from build123d import *

# Parameters (mm, degrees)
SKETCH1_W           = 38.1
SKETCH1_H           = 63.5
BOSS_EXTRUDE1_DEPTH = 36.5125
SKETCH2_W           = 34.925
SKETCH2_H           = 39.6875
CUT_EXTRUDE1_DEPTH  = 62.585998054
SKETCH3_R           = 4.445
CUT_EXTRUDE2_DEPTH  = 76.685633751
SKETCH4_R           = 11.684
CUT_EXTRUDE3_DEPTH  = 6.35
SKETCH6_R           = 14.2621
CUT_EXTRUDE5_DEPTH  = 6.35
SKETCH7_R           = 7.62
CUT_EXTRUDE6_DEPTH  = 71.44279705


with BuildPart() as part:
    # Sketch1 → Boss-Extrude1 (new, symmetric)
    with BuildSketch(Plane.XY):
        Rectangle(SKETCH1_W, SKETCH1_H)
    extrude(amount=BOSS_EXTRUDE1_DEPTH, both=True)

    # Sketch2 → Cut-Extrude1 (cut, through all)
    with BuildSketch(Plane(origin=(19.05, 0, 0), x_dir=(0, 0, -1), z_dir=(1, 0, 0))):
        with Locations((-19.05, 0)):
            Rectangle(SKETCH2_W, SKETCH2_H)
    extrude(amount=-CUT_EXTRUDE1_DEPTH, mode=Mode.SUBTRACT)

    # Sketch3 → Cut-Extrude2 (cut, through all)
    with BuildSketch(Plane(origin=(0, 31.75, 0), x_dir=(1, 0, 0), z_dir=(0, 1, 0))):
        with Locations(Location((0, -20.6375, 0), (0, 0, 270))):
            Circle(SKETCH3_R)
    extrude(amount=-CUT_EXTRUDE2_DEPTH, mode=Mode.SUBTRACT)

    # Sketch4 → Cut-Extrude3 (cut)
    with BuildSketch(Plane(origin=(0, 31.75, 0), x_dir=(1, 0, 0), z_dir=(0, 1, 0))):
        with Locations(Location((0, -20.6375, 0), (0, 0, 270))):
            Circle(SKETCH4_R)
    cut_extrude3 = extrude(amount=-CUT_EXTRUDE3_DEPTH, mode=Mode.SUBTRACT)

    # Sketch6 → Cut-Extrude5 (cut)
    with BuildSketch(Plane(origin=(0, 31.75, 0), x_dir=(1, 0, 0), z_dir=(0, 1, 0))):
        with Locations(Location((0, 20.9296, 0), (0, 0, 270))):
            Circle(SKETCH6_R)
    cut_extrude5 = extrude(amount=-CUT_EXTRUDE5_DEPTH, mode=Mode.SUBTRACT)

    # Mirror1: Cut-Extrude3, Cut-Extrude5 across plane
    add(cut_extrude3.mirror(Plane.ZX), mode=Mode.SUBTRACT)
    add(cut_extrude5.mirror(Plane.ZX), mode=Mode.SUBTRACT)

    # Sketch7 → Cut-Extrude6 (cut, through all)
    with BuildSketch(Plane(origin=(0, 25.4, 0), x_dir=(1, 0, 0), z_dir=(0, 1, 0))):
        with Locations(Location((0, 20.9296, 0), (0, 0, 270))):
            Circle(SKETCH7_R)
    extrude(amount=-CUT_EXTRUDE6_DEPTH, mode=Mode.SUBTRACT)


solid = part.part
CAD build for the part. Positions are in the model's coordinates, mm. A direction names the side the tool comes from. Give positions to 0.01 mm unless a question says otherwise; leave off trailing zeros. Order: outer loops, then holes, each group sorted by start corner. A loop starts at its lowest first (then second) coordinate and runs counter-clockwise, first axis right, second up. Notation, with made-up numbers: (64, 86) - (85, 86) arc R5 cw to (85, 95) - close; hole circle Ø10 at (-19, 65). An arc over 180 degrees is marked (long way). Write each question's results on one line, items separated by ' | '.
1. Saw through at C-C on x = 0. Count the separate pieces of the cut face and the enclosed holes in it, and give its area (3 significant figures).
Calculated:
separate pieces: 4 | enclosed holes: 0 | area: 1,720 mm2
2. Pull direction Y, two halves, no side cores. Call faces 1 (the face through (-0.3, 31.75, 8.6)), 2 (the face through (-8.678, -28.619, -32.248)), 3 (the face through (0, 19.844, 15)): released by +Y, released by -Y, zero draft, split by the parting line, or undercut.
Calculated:
face 1: released by +Y | face 2: zero draft | face 3: undercut
3. Pin check, flat tips, straight feed: pin 1 (14 mm diameter, centred on x = 0, z = 20.64, fed in from +Y); pin 2 (10.5 mm diameter, centred on x = 0.5, z = 18, fed in from -Y); pin 3 (3 mm diameter, centred on x = 9, z = 14, fed in from +Y); pin 4 (12 mm diameter, centred on x = 7, y = -12, fed in from +Z). Stop position of each tip, or through.
Calculated:
pin 1: stops at y = 25.4 | pin 2: stops at y = -25.4 | pin 3: stops at y = 31.75 | pin 4: stops at z = 1.59
4. Probe L1, parallel to Y at x = 2, z = 9; L2, parallel to Y at x = -2.5, z = 31; L3, parallel to Z at x = -9, y = 26. List the from-to ranges inside material, lowest first. Write a range as from..to.
Calculated:
L1: y = -31.75..-19.84, 19.84..31.75 | L2: y = -25.4..-19.84, 19.84..25.4 | L3: z = -36.51..-31.99, -9.87..13.19, 28.09..36.51
5. 3-axis set-ups, long thin cutter, end or side, ignore diameter. For faces 4 (the face through (0, -19.844, 15)), 5 (the face through (-6, 25.4, -15)), 6 (the face through (0, 26, 36.512)), 7 (the face through (-5, -25.4, 20)): which of +Z, -Z, +X, -X, +Y, -Y reach the whole face in a straight line?
Calculated:
face 4: +Z, +X, -X | face 5: +Y | face 6: +Z, +X, -X, +Y, -Y | face 7: -Y
6. Saw through at B-B on y = 8.5. List the corners of the cut face in (x, z).
Calculated:
outline: (-19.05, -36.51) - (19.05, -36.51) - (19.05, 1.59) - (-19.05, 1.59) - close; hole circle Ø15.24 at (0, -20.93)
7. Saw through at A-A on z = 5. List the corners of the cut face in (x, y), and give its area (3 significant figures).
Calculated:
outline: (-19.05, -31.75) - (19.05, -31.75) - (19.05, -19.84) - (-19.05, -19.84) - close; (-19.05, 19.84) - (19.05, 19.84) - (19.05, 31.75) - (-19.05, 31.75) - close | area: 907 mm2
